Autodesk Inventor part; units mm, degrees
ref_plane "YZ Plane" through (0, 0, 0) normal (1, 0, 0) x (0, 1, 0)
ref_plane "XZ Plane" through (0, 0, 0) normal (0, 1, 0) x (-1, 0, 0)
ref_plane "XY Plane" through (0, 0, 0) normal (0, 0, 1) x (1, 0, 0)
sketch "Sketch1" plane through (0, 0, 0) normal (0, 0, 1) x (1, 0, 0)
  circle A0 centre (0, 0) radius 69
  dimension "d0" = 138
extrude "Extrusion1" add sketch "Sketch1" against normal blind 6
sketch "Sketch2" plane through (0, 0, 0) normal (0, 0, 1) x (1, 0, 0)
  circle A0 centre (0, 0) radius 86.0347
extrude "Extrusion2" add sketch "Sketch2" along normal blind 10
sketch "Sketch3" plane through (0, 0, 10) normal (0, 0, 1) x (1, 0, 0)
  circle A0 centre (0, 0) radius 86.0347
  circle A1 centre (0, 0) radius 15.5 construction
  circle A2 centre (0, 15.5) radius 1.75
  circle A3 centre (-15.5, 0) radius 1.75
  circle A4 centre (0, -15.5) radius 1.75
  circle A5 centre (15.5, 0) radius 1.75
  dimension "d5" = 31
  dimension "d6" = 3.5
  dimension "d9" = 360
extrude "Extrusion3" cut sketch "Sketch3" against normal through all contours A2 | A3 | A4 | A5
sketch "Sketch4" plane through (0, 0, 10) normal (0, 0, 1) x (1, 0, 0)
  circle A0 centre (15.5, 0) radius 1.75
  circle A1 centre (-15.5, 0) radius 1.75
  circle A2 centre (0, -15.5) radius 1.75
  circle A3 centre (0, 15.5) radius 1.75
  circle A4 centre (0, 0) radius 86.0347
  circle A5 centre (0, -15.5) radius 3
  circle A6 centre (15.5, 0) radius 3
  circle A7 centre (0, 15.5) radius 3
  circle A8 centre (-15.5, 0) radius 3
  dimension "d13" = 6
  dimension "d16" = 360
extrude "Extrusion4" cut sketch "Sketch4" against normal blind 1 contours A0 | A1 | A3 | A5 | A6 | A7 | A8
sketch "Sketch5" plane through (0, 0, 0) normal (1, 0, 0) x (0, 1, 0)
  line L0 (86.0347, 10) -> (-86.0347, 10)
  line L1 (-86.0347, 0) -> (-86.0347, 10)
  line L2 (0, 0) -> (0, 58.0565)
  line L3 (-22.0852, 10) -> (-23.5623, 10) construction
  line L4 (-23.5623, 10) -> (-67.5613, 8.2465) construction
  line L5 (-67.5613, 8.2465) -> (-86.0347, 1.135) construction
  spline S0 degree 3 poles (-22.0852, 10) (-23.5623, 10) (-67.5613, 8.2465) (-86.0347, 1.135) knots 1 1 1 1 2 2 2 2
revolve "Revolution1" [suppressed]
sketch "Sketch6" plane through (0, 0, -6) normal (0, 0, -1) x (-1, 0, 0)
  circle A0 centre (-15.5, 0) radius 1.75
  circle A1 centre (15.5, 0) radius 1.75
  circle A2 centre (0, -15.5) radius 1.75
  circle A3 centre (0, 15.5) radius 1.75
  circle A4 centre (0, 0) radius 69
  circle A5 centre (0, 0) radius 64.6782
extrude "Extrusion5" cut sketch "Sketch6" against normal blind 8 contours A5
chamfer "Chamfer1" distance 4 angle 45 1 edges at (-86.0347, 0, 10)
chamfer "Chamfer2" distance 2 angle 45 1 edges at (64.6782, 0, -6)
sketch "Sketch7" plane through (0, 0, 2) normal (0, 0, -1) x (-1, 0, 0)
  circle A0 centre (0, 0) radius 64.6782
  circle A1 centre (0, 15.5) radius 1.75
  circle A2 centre (0, -15.5) radius 1.75
  circle A3 centre (15.5, 0) radius 1.75
  circle A4 centre (-15.5, 0) radius 1.75
extrude "Extrusion6" cut sketch "Sketch7" against normal blind 3
properties part number "hoverboardHubCap" material "ABS Plastic"
Work out the finished part from the listing and answer in its coordinate system (mm). A direction names the side the tool comes from. Coordinates: 2 decimals unless noted, no trailing zeros. Loops run counter-clockwise (first coordinate to the right, second up) from the corner with the lowest first, then second, coordinate; pieces in that order, holes last.
1) Section A-A (z = 2.75) is taken. Give the vertices of the cut face in (x, y).
Results:
outline: circle Ø172.07 at (0, 0); hole circle Ø129.36 at (0, 0)
2) For a pull along Y with two mould halves and no side action, classify faces 1 (the cylindrical face through (-68.274, 52.351, 2.958)), 2 (the flat face through (-64.13, 25.89, 0)), 3 (the flat face through (17.5, 0, 9)) as +Y half, -Y half, draft (parallel to the pull), parting line (faces both ways), or undercut.
Results:
face 1: parting line
face 2: draft
face 3: undercut
3) Flat-ended cylindrical pins translate along their axes: pin 1 (1.5 mm diameter, centred on x = 21, z = 2, fed in from +Y); pin 2 (2 mm diameter, centred on x = 48.5, y = 68, fed in from +Z); pin 3 (5.5 mm diameter, centred on x = 0, y = -15.5, fed in from +Z). Find the tip coordinate at first contact, or state that the pin passes through.
Results:
pin 1: stops at y = 83.62
pin 2: stops at z = 9.51
pin 3: stops at z = 9
4) Consider probe 1 along Y at (x, z) = (0, 1.75); probe 2 along Y at (x, z) = (0, 9.45); probe 3 along Y at (x, z) = (0, 6.45). Determine where each line is inside the solid, lowest interval first.
Results:
probe 1: y = -86.03 to -64.68, 64.68 to 86.03
probe 2: y = -82.58 to -18.5, -12.5 to 12.5, 18.5 to 82.58
probe 3: y = -85.58 to -17.25, -13.75 to 13.75, 17.25 to 85.58
5) For faces 4 (the cylindrical face through (12.5, 0.1, 9.5)), 5 (the flat face through (-36, 57, -6)), 6 (the flat face through (1, 1, 5)), determine the directions among +Z, -Z, +X, -X, +Y, -Y from which every point of the face is accessible in a straight line to the end or side of a thin tool.
Results:
face 4: +Z
face 5: -Z, +X, -X, +Y, -Y
face 6: -Z
